from build123d import *

# Parameters (mm, degrees)
BASPROSKE_W              = 4
BASPROSKE_H              = 14
TOOTHCUT_DEPTH           = 21.199009877
TEETHCUTS_COUNT          = 12
TEETHCUTS_ANGLE          = 330
BORSKE_R                 = 4
BORE_DEPTH               = 50.0000508
EXTRUDE_1_DEPTH          = 4
FILLET_1_R               = 10
EXTRUDE_2_DEPTH          = 15
FILLET_2_R               = 2
FILLET_3_R               = 10
EXTRUDE_START            = -4
SKETCH_6_R               = 4
SKETCH_6_R_2             = 1.4
EXTRUDE_3_DEPTH          = 4
CUT_EXTRUDE_6_DEPTH      = 15
CUT_EXTRUDE_6_DEPTH_BACK = 34
SKETCH_7_R               = 1.4
SKETCH_8_R               = 3
CUT_EXTRUDE_7_DEPTH      = 6
SKETCH_10_R              = 1.4
CUT_EXTRUDE_8_DEPTH      = 15


with BuildPart() as part:
    # BasProSke → Base-Revolve (revolve)
    with BuildSketch(Plane(origin=(0, 0, 0), x_dir=(1, 0, 0), z_dir=(0, 1, 0)), mode=Mode.PRIVATE) as base_revolve_sk:
        with Locations((2, 7)):
            Rectangle(BASPROSKE_W, BASPROSKE_H)
    revolve(base_revolve_sk.sketch.rotate(Axis((-10, 0, 0), (1, 0, 0)), 180), axis=Axis((-10, 0, 0), (1, 0, 0)))

    # TooCutSke → ToothCut (cut, through all)
    with BuildSketch(Plane(origin=(0, 0, 0), x_dir=(0, 0, -1), z_dir=(1, 0, 0))):
        with BuildLine():
            ThreePointArc((1.286803432, 9.41143655), (0, 9.499), (-1.286803432, 9.41143655))
            ThreePointArc((-1.286803432, 9.41143655), (-1.63841703, 11.778122922), (-3.088844097, 13.681041163))
            ThreePointArc((-3.088844097, 13.681041163), (0, 14.0254), (3.088844097, 13.681041163))
            ThreePointArc((3.088844097, 13.681041163), (1.63841703, 11.778122922), (1.286803432, 9.41143655))
        make_face()
    toothcut = extrude(amount=TOOTHCUT_DEPTH, mode=Mode.SUBTRACT)

    # TeethCuts: ToothCut ×12 about axis
    teethcuts_axis = Axis((-10, 0, 0), (1, 0, 0))
    for i in range(1, TEETHCUTS_COUNT):
        add(toothcut.rotate(teethcuts_axis, i * TEETHCUTS_ANGLE / (TEETHCUTS_COUNT - 1)), mode=Mode.SUBTRACT)

    # BorSke → Bore (cut, symmetric)
    with BuildSketch(Plane(origin=(0, 0, 0), x_dir=(0, 0, -1), z_dir=(1, 0, 0))):
        with Locations(Location((0, 0, 0), (0, 0, 180))):
            Circle(BORSKE_R)
    extrude(amount=BORE_DEPTH, both=True, mode=Mode.SUBTRACT)

    # 草图3 → 凸台-拉伸1 (add)
    with BuildSketch(Plane(origin=(4, 0, 0), x_dir=(0, 0, -1), z_dir=(1, 0, 0))):
        with BuildLine():
            Line((-0.932792576, -9.484020621), (-7.220100828, -13.585142245))
            Line((-7.220100828, -13.585142245), (-17.903981346, -4.642128436))
            Line((-17.903981346, -4.642128436), (-27.107817182, 27.455461598))
            Line((-27.107817182, 27.455461598), (-31.27472335, 41.987190356))
            Line((-31.27472335, 41.987190356), (-32.818773393, 47.371932777))
            Line((-32.818773393, 47.371932777), (-19.769712012, 64.746456846))
            Line((-19.769712012, 64.746456846), (-10.953080107, 72.951947941))
            Line((-10.953080107, 72.951947941), (-6.126084714, 56.118214487))
            Line((-6.126084714, 56.118214487), (-5.836675561, 55.108924829))
            ThreePointArc((-5.836675561, 55.108924829), (-15.58167252, 49.050779668), (-18.188670428, 37.876270712))
            Line((-18.188670428, 37.876270712), (-11.502054977, 37.992325671))
            Line((-11.502054977, 37.992325671), (-11.26200008, 37.155154756))
            Line((-11.26200008, 37.155154756), (-16.947814294, 33.548891109))
            Line((-16.947814294, 33.548891109), (-16.509005291, 32.018582252))
            Line((-16.509005291, 32.018582252), (-9.82238984, 32.134637212))
            Line((-9.82238984, 32.134637212), (-9.582334943, 31.297466297))
            Line((-9.582334943, 31.297466297), (-15.268149157, 27.691202649))
            Line((-15.268149157, 27.691202649), (-14.829340154, 26.160893793))
            Line((-14.829340154, 26.160893793), (-8.142724703, 26.276948752))
            Line((-8.142724703, 26.276948752), (-7.902669806, 25.439777837))
            Line((-7.902669806, 25.439777837), (-13.58848402, 21.83351419))
            Line((-13.58848402, 21.83351419), (-13.149675017, 20.303205333))
            Line((-13.149675017, 20.303205333), (-6.463059566, 20.419260292))
            Line((-6.463059566, 20.419260292), (-6.223004669, 19.582089377))
            Line((-6.223004669, 19.582089377), (-11.908818883, 15.97582573))
            Line((-11.908818883, 15.97582573), (-5.780671989, 7.422544069))
            ThreePointArc((-5.780671989, 7.422544069), (-4.284008868, -1.296630558), (-0.932792576, -9.484020621))
        make_face()
    extrude(amount=-EXTRUDE_1_DEPTH)

    # 圆角1
    # the kernel refuses this fillet: 10 mm, written as the material it takes off along each edge
    with BuildSketch(Plane(origin=(16.439550253, 47.371932777, 32.818773393), x_dir=(0, 0.7995984784044031, -0.6005349892665399), z_dir=(-1, 0, 0))) as fillet_1_piece_1:
        with BuildLine():
            CenterArc((FILLET_1_R * 0.497582010116, FILLET_1_R), FILLET_1_R, 217.091776954, 52.908223046)
            Line((-FILLET_1_R * 0.300088482439, FILLET_1_R * 0.396906487096), (-FILLET_1_R * 0.31604189229, FILLET_1_R * 0.384844616838))
            Line((-FILLET_1_R * 0.31604189229, FILLET_1_R * 0.384844616838), (-FILLET_1_R * 0.00995164020233, -FILLET_1_R * 0.02))
            Line((-FILLET_1_R * 0.00995164020233, -FILLET_1_R * 0.02), (FILLET_1_R * 0.497582010116, -FILLET_1_R * 0.02))
            Line((FILLET_1_R * 0.497582010116, -FILLET_1_R * 0.02), (FILLET_1_R * 0.497582010116, 0))
        make_face()
    extrude(amount=28.879100506, mode=Mode.SUBTRACT)
    with BuildSketch(Plane(origin=(6.219749224, 64.746456846, 19.769712012), x_dir=(0, 0.6812807658980115, -0.7320222114235461), z_dir=(-1, 0, 0))) as fillet_1_piece_2:
        with BuildLine():
            CenterArc((FILLET_1_R * 0.0887899689748, FILLET_1_R), FILLET_1_R, 259.852030904, 10.147969096)
            Line((-FILLET_1_R * 0.0874009400017, FILLET_1_R * 0.0156439853417), (-FILLET_1_R * 0.0909247581812, -FILLET_1_R * 0.00404313495151))
            Line((-FILLET_1_R * 0.0909247581812, -FILLET_1_R * 0.00404313495151), (-FILLET_1_R * 0.0017757993795, -FILLET_1_R * 0.02))
            Line((-FILLET_1_R * 0.0017757993795, -FILLET_1_R * 0.02), (FILLET_1_R * 0.0887899689748, -FILLET_1_R * 0.02))
            Line((FILLET_1_R * 0.0887899689748, -FILLET_1_R * 0.02), (FILLET_1_R * 0.0887899689748, 0))
        make_face()
    extrude(amount=8.439498449, mode=Mode.SUBTRACT)
    with BuildSketch(Plane(origin=(11.659672741, -4.642128436, 17.903981346), x_dir=(0, 0.9612616959383188, 0.2756373558169997), z_dir=(-1, 0, 0))) as fillet_1_piece_3:
        with BuildLine():
            CenterArc((FILLET_1_R * 0.306386909629, FILLET_1_R), FILLET_1_R, 235.931242449, 34.068757551)
            Line((-FILLET_1_R * 0.253800473888, FILLET_1_R * 0.171634081249), (-FILLET_1_R * 0.265004221559, FILLET_1_R * 0.155066762874))
            Line((-FILLET_1_R * 0.265004221559, FILLET_1_R * 0.155066762874), (-FILLET_1_R * 0.00612773819259, -FILLET_1_R * 0.02))
            Line((-FILLET_1_R * 0.00612773819259, -FILLET_1_R * 0.02), (FILLET_1_R * 0.306386909629, -FILLET_1_R * 0.02))
            Line((FILLET_1_R * 0.306386909629, -FILLET_1_R * 0.02), (FILLET_1_R * 0.306386909629, 0))
        make_face()
    extrude(amount=19.319345481, mode=Mode.SUBTRACT)
    with BuildSketch(Plane(origin=(19.737715423, -13.585142245, 7.220100828), x_dir=(0, 0.6418678587609061, 0.7668152658167999), z_dir=(-1, 0, 0))) as fillet_1_piece_4_section:
        with BuildLine():
            CenterArc((6.295086169, 10), FILLET_1_R, 223.606014756, 46.393985244)
            Line((-0.945908461, 3.103044385), (-1.090728354, 2.965105272))
            ThreePointArc((-1.090728354, 2.965105272), (-0.664263166, 1.493205031), (-0.191308935, -0.058317161))
            Line((-0.191308935, -0.058317161), (0, -0.2))
            Line((0, -0.2), (6.295086169, -0.2))
            Line((6.295086169, -0.2), (6.295086169, 0))
        make_face()
    fillet_1_piece_4 = extrude(amount=35.475430846, mode=Mode.PRIVATE)
    fillet_1_piece_4 = fillet_1_piece_4 - Plane(origin=(2, -11.614079795, -0.29286421), x_dir=(0, 0.587528112701377, 0.8092037548019401), z_dir=(-1, 0, 0)) * Cylinder(4.8, 97, mode=Mode.PRIVATE)
    add(fillet_1_piece_4, mode=Mode.SUBTRACT)

    # 草图4 → 凸台-拉伸2 (add)
    with BuildSketch(Plane(origin=(4, 0, 0), x_dir=(0, 0, -1), z_dir=(1, 0, 0))):
        Polygon((-13.512013594, 70.700072728), (-8.828756529, 54.367614394), (-5.828756529, 55.138253385), (-10.945161074, 72.981276497), align=None)
    extrude(amount=-EXTRUDE_2_DEPTH)

    # 圆角2
    fillet_2_edges = [part.edges().sort_by_distance(p)[0] for p in [
        (-3.5, 72.981276497, 10.945161074),
    ]]
    fillet(fillet_2_edges, radius=FILLET_2_R)

    # 圆角3
    fillet_3_edges = [part.edges().sort_by_distance(p)[0] for p in [
        (0, 62.482661808, 11.15570893),
    ]]
    fillet(fillet_3_edges, radius=FILLET_3_R)

    # 草图6 → 凸台-拉伸3 (add)
    with BuildSketch(Plane.ZY.offset(EXTRUDE_START)):
        Circle(SKETCH_6_R)
        Circle(SKETCH_6_R_2, mode=Mode.SUBTRACT)
    extrude(amount=EXTRUDE_3_DEPTH)

    # 草图7 → 切除-拉伸6 (cut, two sides: drawn at the far end of the back side and taken through both)
    with BuildSketch(Plane(origin=(0, 2.640469614, -9.20841187), x_dir=(-1, 0, 0), z_dir=(0, 0.275637355817, -0.9612616959383188)).offset(-CUT_EXTRUDE_6_DEPTH_BACK)):
        with Locations(Location((4, 62.608913997, 0), (0, 0, 90))):
            Circle(SKETCH_7_R)
    extrude(amount=CUT_EXTRUDE_6_DEPTH + CUT_EXTRUDE_6_DEPTH_BACK, mode=Mode.SUBTRACT)

    # 草图8 → 切除-拉伸7 (cut)
    with BuildSketch(Plane(origin=(0, 1.791367175, -6.247239762), x_dir=(1, 0, 0), z_dir=(0, -0.275637355817, 0.9612616959383187))):
        with Locations(Location((-4, 62.608913997, 0), (0, 0, 90))):
            Circle(SKETCH_8_R)
    extrude(amount=CUT_EXTRUDE_7_DEPTH, mode=Mode.SUBTRACT)

    # 草图10 → 切除-拉伸8 (cut)
    with BuildSketch(Plane(origin=(4, 0, 0), x_dir=(0, 0, -1), z_dir=(1, 0, 0))):
        with Locations((-25.423875567, 43.350590959)):
            Circle(SKETCH_10_R)
        with Locations((-21.28931523, 28.93166552)):
            Circle(SKETCH_10_R)
        with Locations((-17.154754893, 14.512740081)):
            Circle(SKETCH_10_R)
        with Locations((-13.020194555, 0.093814642)):
            Circle(SKETCH_10_R)
    extrude(amount=-CUT_EXTRUDE_8_DEPTH, mode=Mode.SUBTRACT)


solid = part.part
The listing builds one solid part. Answer for the finished solid, in the listing's coordinates (mm). Round coordinates to 2 decimals unless told otherwise and drop trailing zeros. Write each loop counter-clockwise with the first axis right and the second up, starting at its lowest first coordinate (ties: lowest second). Pieces come first, ordered by that corner, then holes. Notation, with made-up numbers: M 53.5,-31.75 L 78.5,-31.75 A24 cw 78.5,7.25 Z; hole C 32.25,66 d5. An arc over 180 degrees is marked long. Write each question's results on one line, items separated by ' | '. Start each with the question number.
Item 1: Given pin 1 Ø4.5 at (y, z) = (0.09, 13.02) entering from -X; pin 2 Ø2.5 at (y, z) = (28.93, 21.29) entering from -X; pin 3 Ø6 at (x, y) = (1.5, 11) entering from -Z; pin 4 Ø2 at (x, y) = (1.5, 31.5) entering from +Z, each flat-ended and moving along its own axis, determine where each tip first touches the part or whether it passes through.
Item 2: Find section B-B on y = 48.5. Write down the section's boundary in (x, z).
Item 3: Straight lines are drawn through the part: probe 1 along X at (y, z) = (26.5, 17); probe 2 along Y at (x, z) = (2, 3.5); probe 3 along Y at (x, z) = (-5.75, 12.5). For each, find the intervals that lie inside material, in ascending order.
Item 4: Find section A-A on z = 0. Write down the section's boundary in (x, y), and give its area (3 significant figures).
Item 5: The mould has two halves that part along Z. Classify faces 1 (the flat face through (2.03, 17.8, 9.03)), 2 (the flat face through (0.209, 68.521, 15.714)), 3 (the cylindrical face through (2, 9.5, 0)): +Z half, -Z half, draft (parallel to the pull), parting line (faces both ways), or undercut.
Answer block:
1) pin 1: stops at x = 0 | pin 2: passes through | pin 3: stops at z = -10.3 | pin 4: stops at z = 28.55
2) outline: M 0,15.96 L 4,15.96 L 4,31.32 L 0,31.32 Z
3) probe 1: x = 0 to 4 | probe 2: y = -13.56 to 13.56 | probe 3: y = 64.08 to 71.31
4) outline: M 0,-9.5 L 4,-9.5 L 4,-1.4 L 0,-1.4 Z; M 0,1.4 L 4,1.4 L 4,9.5 L 0,9.5 Z | area: 64.8 mm²
5) face 1: -Z half | face 2: +Z half | face 3: undercut
